Here's the drawing with two shaded views (mm, measured from the low corner). I have some questions. Coordinates: 2 decimals unless noted, no trailing zeros. Loops run counter-clockwise (first coordinate to the right, second up) from the corner with the lowest first, then second, coordinate; pieces in that order, holes last.
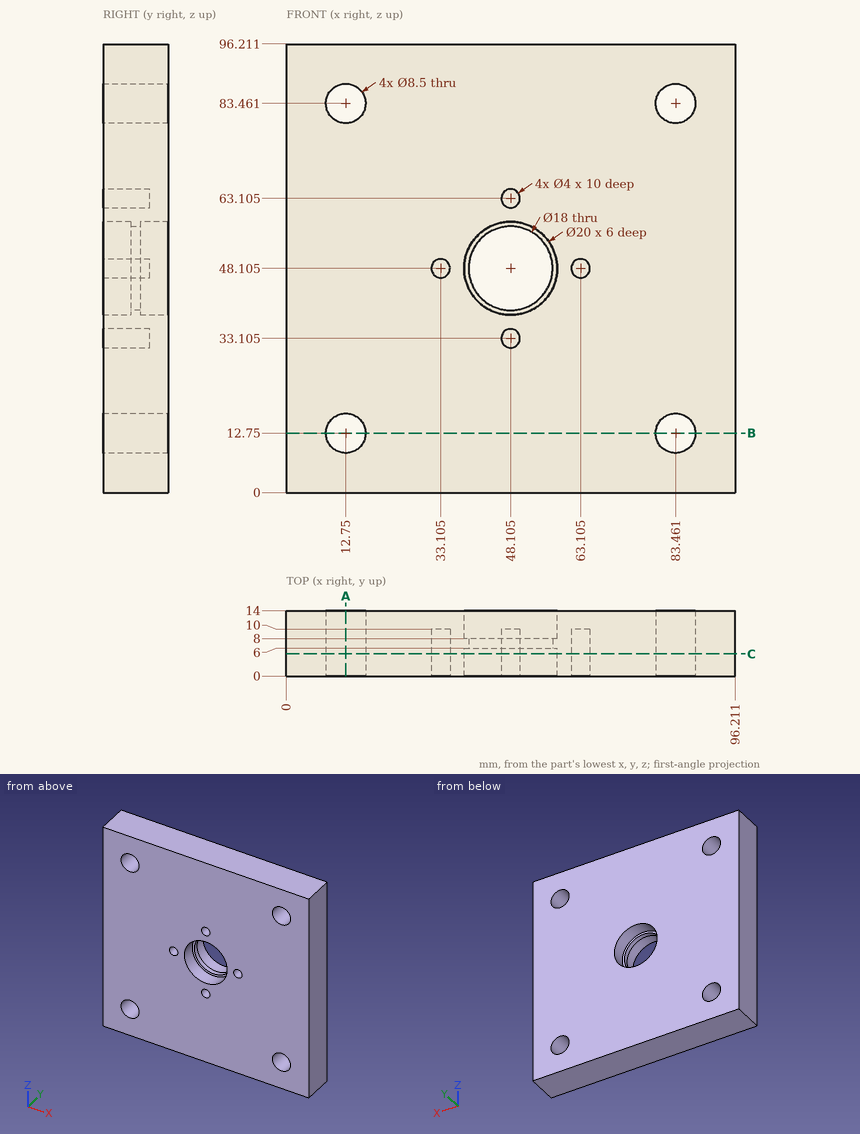
(1) I want a section at C-C on y = 4.75. State how many separate pieces and enclosed holes the cut face has.
Check values:
separate pieces: 1
enclosed holes: 9
(2) I want a section at A-A on x = 12.75. Write out the boundary of the cut face in (y, z).
Check values:
outline: (0, 0) - (14, 0) - (14, 8.5) - (0, 8.5) - close; (0, 17) - (14, 17) - (14, 79.21) - (0, 79.21) - close; (0, 87.71) - (14, 87.71) - (14, 96.21) - (0, 96.21) - close
(3) I'm going to push flat-ended pins straight in: pin 1 (12 mm diameter, centred on x = 60.5, z = 32, fed in from -Y); pin 2 (11 mm diameter, centred on x = 48.11, z = 48.11, fed in from +Y); pin 3 (1.2 mm diameter, centred on x = 63, z = 48, fed in from -Y). Where does each tip first touch, or does it pass through?
Check values:
pin 1: stops at y = 0
pin 2: passes through
pin 3: stops at y = 10
(4) If I drill on probe 1 along Z at (x, y) = (48, 4.5) (1 decimal); probe 2 along X at (y, z) = (6.5, 48) (1 decimal); probe 3 along Z at (x, y) = (14, 11.5), over which ranges is the centre line in solid material (lowest first)?
Check values:
probe 1: z = 0 to 31.1, 35.1 to 38.1, 58.1 to 61.1, 65.1 to 96.2
probe 2: x = 0 to 31.1, 35.1 to 39.1, 57.1 to 61.1, 65.1 to 96.2
probe 3: z = 0 to 8.69, 16.81 to 79.4, 87.52 to 96.21
(5) I want a section at B-B on z = 12.75. Write out the boundary of the cut face in (x, y).
Check values:
outline: (0, 0) - (8.5, 0) - (8.5, 14) - (0, 14) - close; (17, 0) - (79.21, 0) - (79.21, 14) - (17, 14) - close; (87.71, 0) - (96.21, 0) - (96.21, 14) - (87.71, 14) - close
